The drawing under review shows one solid part. Ordinate dimensions are in mm from its lowest x, y, z. A direction names the side the tool comes from. Round coordinates to 2 decimals unless told otherwise and drop trailing zeros. Loops run counter-clockwise (first coordinate to the right, second up) from the corner with the lowest first, then second, coordinate; pieces in that order, holes last. Notation, with made-up numbers: (5, 86) - (54, 86) arc R31 cw to (54, 114) - close; hole circle Ø6 at (-32.5, 22.25). An arc over 180 degrees is marked (long way). Answer as CSV lines item,"result".
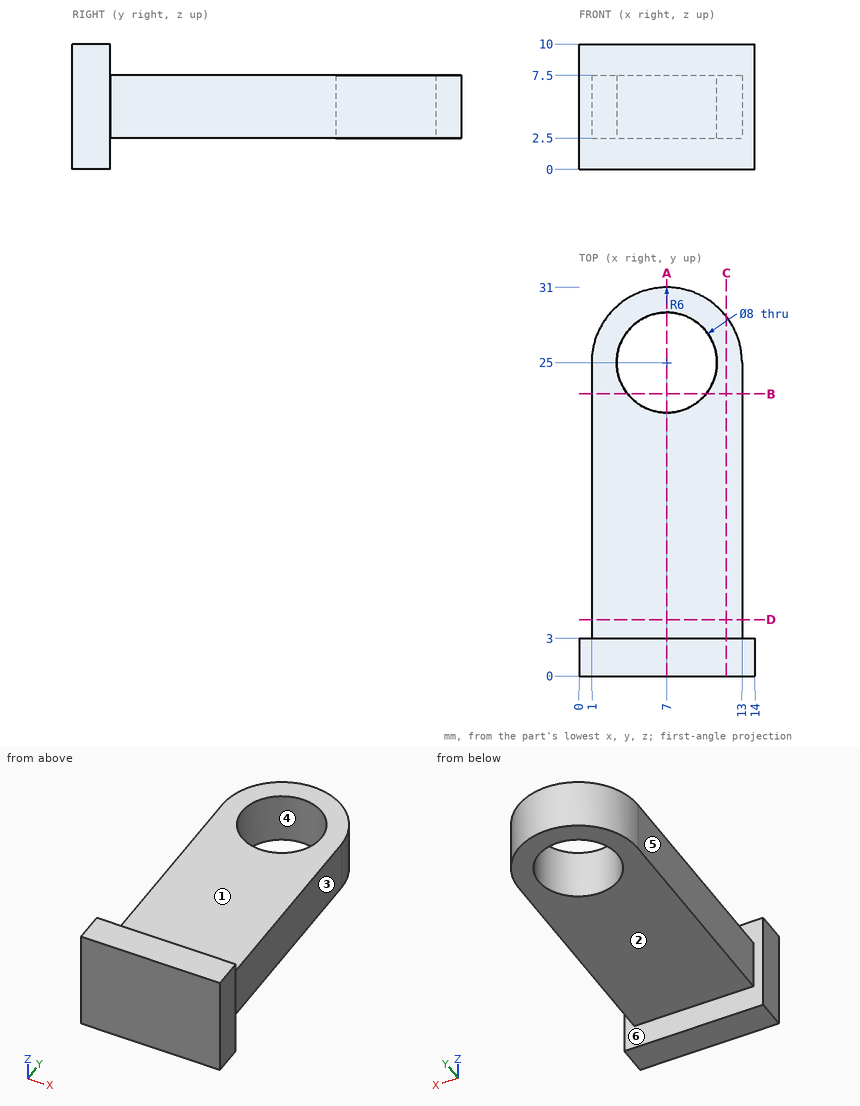
1. Clearance check with flat-ended pins moving along their axes: pin 1 (6 mm diameter, centred on x = 5.5, y = 21.5, fed in from +Z); pin 2 (1.5 mm diameter, centred on y = 11.5, z = 4.5, fed in from -X); pin 3 (2.5 mm diameter, centred on y = 19, z = 6, fed in from +X). State where each tip first meets the part, or that it passes through.
Numbers:
pin 1,"stops at z = 7.5"
pin 2,"stops at x = 1"
pin 3,"stops at x = 13"
2. Take a section at B-B (y = 22.5). State the section outline as (x, z) points, plus the area to 3 significant figures.
Numbers:
outline,"(1, 2.5) - (3.88, 2.5) - (3.88, 7.5) - (1, 7.5) - close; (10.12, 2.5) - (13, 2.5) - (13, 7.5) - (10.12, 7.5) - close"
area,"28.8 mm²"
3. Tool access review of the marked faces 1, 2 and 3: name each direction out of +Z, -Z, +X, -X, +Y, -Y from which nothing blocks a thin tool from reaching the whole face with its end or side.
Numbers:
face 1,"+Z, +X, -X, +Y"
face 2,"-Z, +X, -X, +Y"
face 3,"+Z, -Z, +X, +Y"
4. Take a section at D-D (y = 4.5). State the section outline as (x, z) points, plus the area to 3 significant figures.
Numbers:
outline,"(1, 2.5) - (13, 2.5) - (13, 7.5) - (1, 7.5) - close"
area,"60.0 mm²"
5. Take a section at A-A (x = 7). State the section outline as (y, z) points, plus the area to 3 significant figures.
Numbers:
outline,"(0, 0) - (3, 0) - (3, 2.5) - (21, 2.5) - (21, 7.5) - (3, 7.5) - (3, 10) - (0, 10) - close; (29, 2.5) - (31, 2.5) - (31, 7.5) - (29, 7.5) - close"
area,"130 mm²"
6. Draft analysis for pull direction X (two halves, no side actions). For the marked faces 4, 5 and 6, state which applies: +X half, -X half, draft (parallel to the pull), parting line (faces both ways), or undercut.
Numbers:
face 4,"undercut"
face 5,"-X half"
face 6,"draft"
7. Take a section at C-C (x = 11.75). State the section outline as (y, z) points, plus the area to 3 significant figures.
Numbers:
outline,"(0, 0) - (3, 0) - (3, 2.5) - (28.67, 2.5) - (28.67, 7.5) - (3, 7.5) - (3, 10) - (0, 10) - close"
area,"158 mm²"
8. Wall thickness on probe 1 along Y at (x, z) = (7, 3.7); probe 2 along X at (y, z) = (25, 6); probe 3 along Z at (x, y) = (11.75, 17.5): over which ranges is each line inside the solid? List them lowest first.
Numbers:
probe 1,"y = 0 to 21, 29 to 31"
probe 2,"x = 1 to 3, 11 to 13"
probe 3,"z = 2.5 to 7.5"
